Autodesk Inventor part; units mm, degrees
ref_plane "Work Plane1" through (0, -2.4764, 0) normal (-1, 0, 0) x (0, 0, 1)
ref_plane "YZ Plane" through (0, 0, 0) normal (1, 0, 0) x (0, 1, 0)
ref_plane "XZ Plane" through (0, 0, 0) normal (0, 1, 0) x (-1, 0, 0)
sketch "Esquisse1" plane through (0, 0, 0) normal (0, 0, 1) x (1, 0, 0)
  circle A0 centre (0, -2.4764) radius 2.5 construction
  line L0 (-0.3, 0.0236) -> (0, 0.0236) construction
  line L1 (-3.206, 0) -> (3.4858, 0)
  line L2 (-1.3748, -3.0764) -> (1.3748, -3.0764) construction
  arc A1 (-1.4207, -1.9952) -> (-1.3748, -3.0764) centre (0, -2.4764) ccw
  line L3 (0, 1.949) -> (0, -3.4788)
  arc A2 (-0.3, -0.6764) -> (0.3, -0.6764) centre (0, -0.6764) ccw
  arc A3 (2.6558, -4.756) -> (-2.6558, -4.756) centre (0, -2.4764) ccw
  line L4 (-1.8, -1.8764) -> (-1.506, -1.8764)
  line L5 (-0.3, -0.6764) -> (-0.3, -0.3849)
  arc A4 (-0.6, -0.1526) -> (-2.1176, -1.3469) centre (0, -2.4764) ccw
  arc A5 (-0.3, -0.3849) -> (-0.6, -0.1526) centre (-0.54, -0.3849) ccw
  arc A6 (-2.1176, -1.3469) -> (-1.8, -1.8764) centre (-1.8, -1.5164) ccw
  arc A7 (-1.4207, -1.9952) -> (-1.506, -1.8764) centre (-1.506, -1.9664) ccw
  line L6 (0, 1.0236) -> (2.5298, 1.0236) construction
  line L7 (-1.3748, -3.0764) -> (-1.8877, -4.606)
  arc A8 (-2.6558, -4.756) -> (-1.8877, -4.606) centre (-2.3143, -4.4629) ccw
  line L8 (0, -0.9764) -> (-1.2778, -0.9764) construction
  line L9 (1.3748, -3.0764) -> (1.8877, -4.606)
  arc A9 (1.8877, -4.606) -> (2.6558, -4.756) centre (2.3143, -4.4629) ccw
  arc A10 (1.3748, -3.0764) -> (1.4207, -1.9952) centre (0, -2.4764) ccw
  line L10 (1.8, -1.8764) -> (1.506, -1.8764)
  line L11 (0.3, -0.6764) -> (0.3, -0.3849)
  arc A11 (2.1176, -1.3469) -> (0.6, -0.1526) centre (0, -2.4764) ccw
  arc A12 (0.6, -0.1526) -> (0.3, -0.3849) centre (0.54, -0.3849) ccw
  arc A13 (1.8, -1.8764) -> (2.1176, -1.3469) centre (1.8, -1.5164) ccw
  arc A14 (1.506, -1.8764) -> (1.4207, -1.9952) centre (1.506, -1.9664) ccw
  point P0 (0.3, 0.0236)
  dimension "d0" = 5
  dimension "d3" = 0.6
  dimension "d4" = 0.3
  dimension "d5" = 7
  dimension "d8" = 2.4
  dimension "d9" = 0.6
  dimension "d10" = 0.24
  dimension "d11" = 0.36
  dimension "d12" = 0.09
  dimension "d13" = 0.45
  dimension "d14" = 1.5
  dimension "d15" = 1.5
extrude "Corps" add sketch "Esquisse1" along normal blind 0.6
ref_plane "Work Plane1" through (0, -2.4764, 0) normal (-1, 0, 0) x (0, 0, 1)
equation "\"d0\" = WD"
equation "\"d3\" = 0.2 * NND"
equation "\"d4\" = 0.1 * NND"
equation "\"d5\" = SD2"
equation "\"d8\" = 0.8 * NND"
equation "\"d9\" = 0.2 * NND"
equation "\"d10\" = 0.08 * NND"
equation "\"d11\" = 0.12 * NND"
equation "\"d12\" = 0.03 * NND"
equation "\"d13\" = 0.15 * NND"
equation "\"d14\" = 0.5 * NND"
equation "\"d15\" = 0.5 * NND"
equation "\"d16\" = SD"
equation "\"ND\" = 3.05"
equation "\"SD\" = 0.6"
equation "\"WD\" = 5"
equation "\"d1\" = 1.6 * NND"
equation "\"d2\" = NND"
equation "\"SD2\" = 7"
equation "\"d6\" = NND"
equation "\"d7\" = 0.15 * NND"
equation "\"NND\" = 3"
equation "\"WDMIN\" = 4"
equation "\"SNB\" = 0.7"
equation "\"WDMAX\" = 5"
equation "\"BUBRMI\" = 1"
properties part number "JIS B 2804 E - 3" material "Acier, doux"
Here's how the part is built. I have some questions about the finished solid (model axes, mm). A direction names the side the tool comes from. Coordinates: 2 decimals unless noted, no trailing zeros. Loops run counter-clockwise (first coordinate to the right, second up) from the corner with the lowest first, then second, coordinate; pieces in that order, holes last.
1. Imagine slicing it at C-C, the plane z = 0.3. Please give me the cut outline in (x, y) (3 decimals).
2. Imagine slicing it at D-D, the plane x = 0. Please give me the cut outline in (y, z), and give its area (3 significant figures).
3. I need wall thicknesses on L1, parallel to X at y = -2.45, z = 0.4; L2, parallel to X at y = -0.6, z = 0.15; L3, parallel to X at y = -3.35, z = 0.2. Which ranges of each line are inside material? Lowest first, please.
4. Imagine slicing it at B-B, the plane x = 2. Please give me the cut outline in (y, z), and give its area (3 significant figures).
5. Imagine slicing it at A-A, the plane y = -3.9. Please give me the cut outline in (x, z).
6. For faces 4 (the flat face through (0, -0.6, 0)), 5 (the cylindrical face through (1.47, -0.58, 0.3)), which set-ups out of +Z, -Z, +X, -X, +Y, -Y let a thin tool reach every point of the face, with its end or its side?
7. If we mould it in two halves opening along Y, with no side actions, what happens to faces 1 (the cylindrical face through (-1.495, -0.599, 0.296)), 2 (the flat face through (0, -0.6, 0.6)), 3 (the cylindrical face through (-0.11, 1.02, 0.3))? For each: pulls with the +Y half, pulls with the -Y half, needs draft (parallel to the pull), parting line crosses it, or undercut.
8. For P1, Ø1, axis at x = 1, y = -3, coming from the -Z side, with a flat end and sliding along its axis, tell me the tip position at first contact or that it passes through.
Taken from the geometry:
1. outline: (-2.656, -4.756) arc R0.45 ccw to (-1.888, -4.606) - (-1.375, -3.076) arc R1.5 cw to (-1.421, -1.995) arc R0.09 ccw to (-1.506, -1.876) - (-1.8, -1.876) arc R0.36 cw to (-2.118, -1.347) arc R2.4 cw to (-0.6, -0.153) arc R0.24 cw to (-0.3, -0.385) - (-0.3, -0.676) arc R0.3 ccw to (0.3, -0.676) - (0.3, -0.385) arc R0.24 cw to (0.6, -0.153) arc R2.4 cw to (2.118, -1.347) arc R0.36 cw to (1.8, -1.876) - (1.506, -1.876) arc R0.09 ccw to (1.421, -1.995) arc R1.5 cw to (1.375, -3.076) - (1.888, -4.606) arc R0.45 ccw to (2.656, -4.756) arc R3.5 ccw (long way) to start
2. outline: (-0.98, 0) - (1.02, 0) - (1.02, 0.6) - (-0.98, 0.6) - close
2. area: 1.20 mm2
3. L1: x = -3.5 to -1.5, 1.5 to 3.5
3. L2: x = -2.95 to -1.5, -0.3 to 0.3, 1.5 to 2.95
3. L3: x = -3.39 to -1.47, 1.47 to 3.39
4. outline: (-4.78, 0) - (-1.82, 0) - (-1.82, 0.6) - (-4.78, 0.6) - close; (-1.15, 0) - (0.4, 0) - (0.4, 0.6) - (-1.15, 0.6) - close
4. area: 2.71 mm2
5. outline: (-3.2, 0) - (-1.65, 0) - (-1.65, 0.6) - (-3.2, 0.6) - close; (1.65, 0) - (3.2, 0) - (3.2, 0.6) - (1.65, 0.6) - close
6. face 4: -Z, +X, -X, +Y, -Y
6. face 5: +Z, -Z
7. face 1: undercut
7. face 2: needs draft
7. face 3: parting line crosses it
8. P1: stops at z = 0
